```python
from build123d import *

# Parameters (mm, degrees)
CYLINDER093_R     = 1.5
CYLINDER093_DEPTH = 14
CYLINDER090_R     = 12.5
CYLINDER090_DEPTH = 33
CYLINDER094_R     = 1.5
CYLINDER094_DEPTH = 14
CYLINDER088_R     = 14
CYLINDER088_DEPTH = 33
BOX016_W          = 1
BOX016_H          = 1
BOX016_DEPTH      = 1
CYLINDER084_R     = 17
CYLINDER084_DEPTH = 5


with BuildPart() as obj1:
    # Cylinder093 → Cylinder093 (new body)
    with BuildSketch(Plane(origin=(53.66, 148, -15), x_dir=(1, 0, 0), z_dir=(0, 0, 1))):
        Circle(CYLINDER093_R)
    extrude(amount=CYLINDER093_DEPTH)


with BuildPart() as obj2:
    # Cylinder090 → Cylinder090 (new body)
    with BuildSketch(Plane(origin=(73.66, 148, -10), x_dir=(1, 0, 0), z_dir=(0, 0, 1))):
        Circle(CYLINDER090_R)
    extrude(amount=CYLINDER090_DEPTH)


with BuildPart() as fusion039:
    # Cylinder094 → Cylinder094 (new body)
    with BuildSketch(Plane(origin=(93.66, 148, -14), x_dir=(1, 0, 0), z_dir=(0, 0, 1))):
        Circle(CYLINDER094_R)
    extrude(amount=CYLINDER094_DEPTH)

    # Fusion039: union obj1, obj2
    add(obj1.part)
    add(obj2.part)


with BuildPart() as obj3:
    # Cylinder088 → Cylinder088 (new body)
    with BuildSketch(Plane(origin=(73.66, 148, -10), x_dir=(1, 0, 0), z_dir=(0, 0, 1))):
        Circle(CYLINDER088_R)
    extrude(amount=CYLINDER088_DEPTH)


with BuildPart() as obj4:
    # Box016 → Box016 (new body)
    with BuildSketch(Plane(origin=(63, 136, -8), x_dir=(1, 0, 0), z_dir=(0, 0, 1))):
        with Locations((0.5, 0.5)):
            Rectangle(BOX016_W, BOX016_H)
    extrude(amount=BOX016_DEPTH)


with BuildPart() as obj5:
    # Cylinder084 → Cylinder084 (new body)
    with BuildSketch(Plane(origin=(73.66, 148, -10), x_dir=(1, 0, 0), z_dir=(0, 0, 1))):
        Circle(CYLINDER084_R)
    extrude(amount=CYLINDER084_DEPTH)

    # Fusion038: union obj3, obj4
    add(obj3.part)
    add(obj4.part)

    # Cut010: cut Fusion039
    add(fusion039.part, mode=Mode.SUBTRACT)


with BuildPart() as obj5_1:
    # Cut010 placement: moved
    add(obj5.part.moved(Location((-73.66, -148, -23))))


solid = obj5_1.part
```
Geometry: final body of the model. Coordinates: model frame, mm. Round coordinates to 2 decimals unless told otherwise and drop trailing zeros. Write each loop counter-clockwise with the first axis right and the second up, starting at its lowest first coordinate (ties: lowest second). Pieces come first, ordered by that corner, then holes.
Item 1: Pin query (flat end, axial travel): P1, Ø6, axis at x = 4.5, z = -12.5, coming from the -Y side; P2, Ø2, axis at x = -4.5, y = -10.5, coming from the -Z side; P3, Ø6, axis at x = -3, z = -3.5, coming from the -Y side; P4, Ø3, axis at x = 6.5, z = -17, coming from the +Y side. Return the tip coordinate at first contact, or that it passes through.
Item 2: Material intervals for L1, parallel to Y at x = 0, z = -21; L2, parallel to Y at x = -8.5, z = -1.5; L3, parallel to Z at x = -14.5, y = -2, sorted ascending.
Item 3: Mould query, pull axis Y, two halves, no side actions, for faces 1 (the face through (-6, 13, -28)), 2 (the face through (-2.71, -12.203, -16.731)), 3 (the face through (-10.32, 9.46, -14.2)). Classes: +Y half, -Y half, draft (parallel to the pull), parting line (faces both ways), or undercut.
Item 4: Section query D-D (y = 15). Return loops of the section in (x, z).
Item 5: Section query A-A (x = 0). Return loops of the section in (y, z), plus the area to 3 significant figures.
Item 6: Section query B-B (y = -6.5). Return loops of the section in (x, z).
Item 7: Section query C-C (z = -5). Return loops of the section in (x, y).
Completed:
1. P1: stops at y = -13.92
1. P2: passes through
1. P3: stops at y = -14
1. P4: stops at y = 13.08
2. L1: y = -14 to -12.5, 12.5 to 14
2. L2: y = -11.12 to -9.17, 9.17 to 11.12
2. L3: z = -33 to -28
3. face 1: draft
3. face 2: undercut
3. face 3: parting line
4. outline: (-8, -33) - (8, -33) - (8, -28) - (-8, -28) - close
5. outline: (-17, -33) - (-12.5, -33) - (-12.5, 0) - (-14, 0) - (-14, -28) - (-17, -28) - close; (12.5, -33) - (17, -33) - (17, -28) - (14, -28) - (14, 0) - (12.5, 0) - close
5. area: 129 mm2
6. outline: (-15.71, -33) - (-10.68, -33) - (-10.68, 0) - (-12.4, 0) - (-12.4, -28) - (-15.71, -28) - close; (10.68, -33) - (15.71, -33) - (15.71, -28) - (12.4, -28) - (12.4, 0) - (10.68, 0) - close
7. outline: circle Ø28 at (0, 0); hole circle Ø25 at (0, 0)
